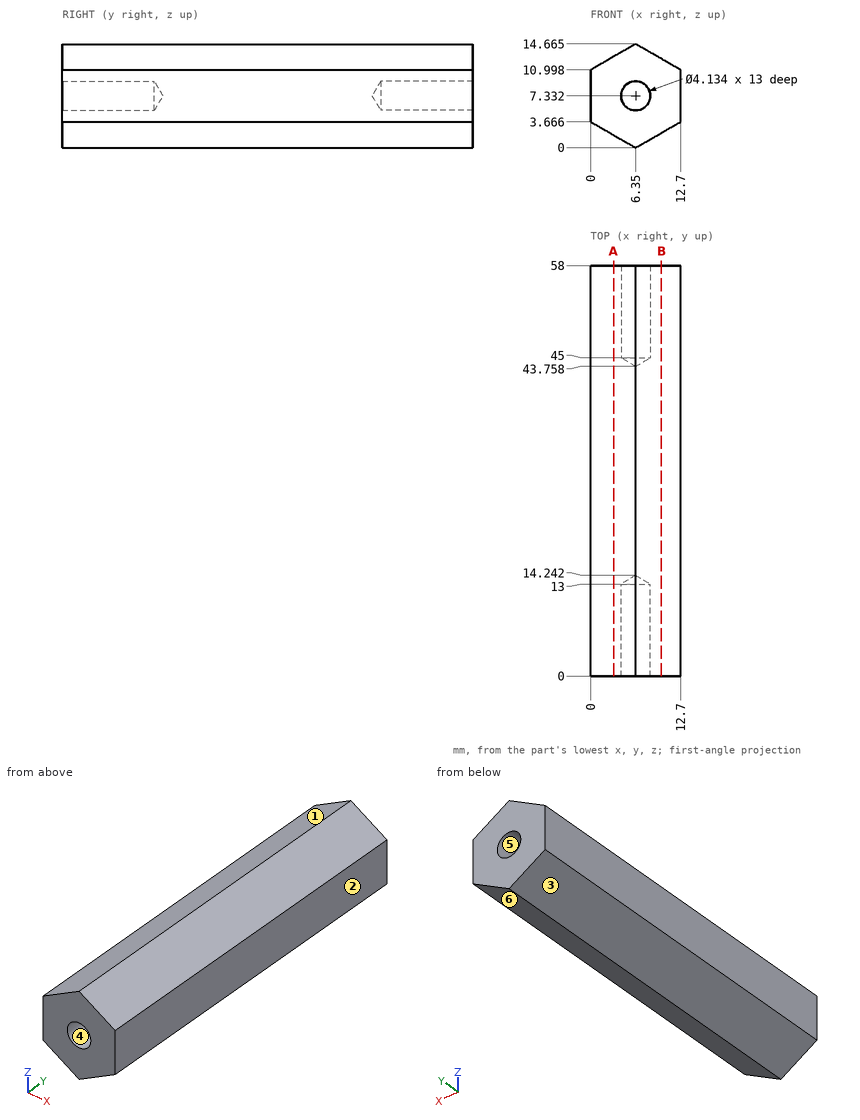
Design review of the part shown in the three views and the two pictorial views. Dimensions are in mm from the part's minimum x, y and z. A direction names the side the tool comes from. Give positions to 0.01 mm unless a question says otherwise; leave off trailing zeros. Loops run counter-clockwise (first coordinate to the right, second up) from the corner with the lowest first, then second, coordinate; pieces in that order, holes last. Notation, with made-up numbers: (57.5, -25.5) - (87.5, -25.5) arc R25 ccw to (87.5, -6.5) - close; hole circle Ø1 at (15.5, -40). An arc over 180 degrees is marked (long way). Write item = value, one per line.
1) Take a section at B-B on x = 10. State the section outline as (y, z) points, and give its area (3 significant figures).
Result sheet:
outline = (0, 2.11) - (58, 2.11) - (58, 12.56) - (0, 12.56) - close
area = 606 mm2
2) Tool access review of the marked faces 5 and 6: name each direction out of +Z, -Z, +X, -X, +Y, -Y from which nothing blocks a thin tool from reaching the whole face with its end or side.
Result sheet:
face_5 = +Y
face_6 = -Z, +X, +Y, -Y
3) Draft analysis for pull direction Z (two halves, no side actions). For the marked faces 1, 2, 3 and 4, state which applies: +Z half, -Z half, draft (parallel to the pull), parting line (faces both ways), or undercut.
Result sheet:
face_1 = +Z half
face_2 = draft
face_3 = -Z half
face_4 = undercut
4) To check wall thickness, follow line 1 (X direction, y = 3, z = 6.75); line 2 (Z direction, x = 5, y = 4.5) (1 decimal); line 3 (Z direction, x = 7, y = 55) (1 decimal). State the ranges of each line that lie inside material, in increasing order.
Result sheet:
line_1 = 0 to 4.37, 8.33 to 12.7
line_2 = 0.8 to 5.8, 8.9 to 13.9
line_3 = 0.4 to 5.4, 9.3 to 14.3
5) Clearance check with flat-ended pins moving along their axes: pin 1 Ø1 at (x, y) = (3, 36.5) entering from +Z; pin 2 Ø1.5 at (x, y) = (3, 6.5) entering from +Z. State where each tip first meets the part, or that it passes through.
Result sheet:
pin_1 = 13.02
pin_2 = 13.16
6) Take a section at A-A on x = 3.25. State the section outline as (y, z) points (1 decimal), and give its area (3 significant figures).
Result sheet:
outline = (0, 1.8) - (58, 1.8) - (58, 12.9) - (0, 12.9) - close
area = 643 mm2
